Part model, mm, in its own coordinate system. A direction names the side the tool comes from. Give positions to 0.01 mm unless a question says otherwise; leave off trailing zeros. Order: outer loops, then holes, each group sorted by start corner. A loop starts at its lowest first (then second) coordinate and runs counter-clockwise, first axis right, second up.
1. Which spindle directions (+Z, -Z, +X, -X, +Y, -Y) get a long thin tool onto all of the face, cutting with end or side? Do faces 1 (the flat face through (0, 0, -12)), 2 (the cylindrical face through (14.2, 3.5, 33.2)), 3 (the flat face through (-12, -1, -44.8)). Say none if no direction does.
2. Slice it at D-D on y = -15.25. List the corners of the cut face in (x, z), and give its area (3 significant figures).
3. Drop flat-ended pins along their axis: pin 1 Ø9.5 at (x, z) = (0, -21.8) entering from -Y; pin 2 Ø5 at (x, z) = (11, 37) entering from -Y; pin 3 Ø3 at (y, z) = (-14, -47) entering from -X; pin 4 Ø4 at (x, y) = (1, -10.5) entering from +Z. Give the stop position or say it passes through.
4. Mould opens along X. For faces 4 (the cylindrical face through (-10.36, 3.52, 38.03)), 5 (the flat face through (12, -1, -44.8)), 6 (the flat face through (31.467, -1, 5)) say: +X half, -X half, draft (parallel to the pull), parting line (faces both ways), or undercut.
5. Slice it at B-B on x = -1.5. List the corners of the cut face in (y, z), and give its area (3 significant figures).
6. Slice it at C-C on x = 17.5. List the corners of the cut face in (y, z).
7. Probe line 1 (X direction, y = -2.1, z = -21.8); line 2 (Y direction, x = 17, z = -35.5); line 3 (Z direction, x = -6.5, y = -1.25). List the from-to ranges inside material, lowest first.
8. Slice it at A-A on z = -21.8. List the corners of the cut face in (x, y), and give its area (3 significant figures).
from build123d import *

# Parameters (mm, degrees)
BASE_FLANGE1_DEPTH           = 3
SKETCH2_R                    = 8
CUT_EXTRUDE1_DEPTH           = 73.112420355
EDGE_FLANGE1_STRIP_W         = 13.4732
EDGE_FLANGE1_STRIP_H         = 3
EDGE_FLANGE1_STRIP_CUT_DEPTH = 62.933077126
EDGE_FLANGE1_DEPTH           = 62.933077126
EDGE_FLANGE2_STRIP_W         = 13.4732
EDGE_FLANGE2_STRIP_H         = 3
EDGE_FLANGE2_STRIP_CUT_DEPTH = 62.933077126
EDGE_FLANGE2_DEPTH           = 62.933077126
CUT_EXTRUDE14_DEPTH          = 73.492766325
CUT_EXTRUDE15_DEPTH          = 73.492766325
CUT_EXTRUDE16_DEPTH          = 73.492766325
SKETCHED_START               = -2.498589927
SKETCHED_BEND2_DEPTH         = 5
SKETCHED_BEND2_2_DEPTH       = 5


# Read off the part's stored shape, not the designer's step: Sketched Bend2
# Sheet-metal steps are written as plain solids
with BuildPart() as part:
    # Sketch1 → Base-Flange1 (new body)
    with BuildSketch(Plane(origin=(0, 0, 0), x_dir=(1, 0, 0), z_dir=(0, 1, 0))):
        with BuildLine():
            Line((2.501410073, 64.8), (-2.498589927, 64.8))
            Line((-2.498589927, 64.8), (-2.498589927, 44.8))
            Line((-2.498589927, 44.8), (-21.498589927, 44.8))
            ThreePointArc((-21.498589927, 44.8), (-28.847059156, 41.582329983), (-31.466538563, 34))
            Line((-31.466538563, 34), (-31.466538563, -26))
            Line((-31.466538563, -26), (31.466538563, -26))
            Line((31.466538563, -26), (31.466538563, 34))
            ThreePointArc((31.466538563, 34), (28.848015597, 41.581293991), (21.501410073, 44.8))
            Line((21.501410073, 44.8), (2.501410073, 44.8))
            Line((2.501410073, 44.8), (2.501410073, 64.8))
        make_face()
    extrude(amount=-BASE_FLANGE1_DEPTH)

    # Sketch2 → Cut-Extrude1 (cut, through all)
    with BuildSketch(Plane(origin=(0, 0, 0), x_dir=(1, 0, 0), z_dir=(0, 1, 0))):
        with Locations(Location((0.000474376, 21.8, 0), (0, 0, 270))):
            Circle(SKETCH2_R)
    extrude(amount=-CUT_EXTRUDE1_DEPTH, mode=Mode.SUBTRACT)

    # Edge-Flange1 strip (across the edge) → Edge-Flange1 strip cut (cut)
    with BuildSketch(Plane(origin=(-31.466538563, 0, 26), x_dir=(0, 0, -1), z_dir=(1, 0, 0))):
        with Locations((-3, -1.5)):
            Rectangle(EDGE_FLANGE1_STRIP_W, EDGE_FLANGE1_STRIP_H)
    extrude(amount=EDGE_FLANGE1_STRIP_CUT_DEPTH, mode=Mode.SUBTRACT)

    # Edge-Flange1 section (across the edge) → Edge-Flange1 (add)
    with BuildSketch(Plane(origin=(-31.466538563, 0, 26), x_dir=(0, 0, -1), z_dir=(1, 0, 0))):
        with BuildLine():
            Line((0, 0.7366), (0, 2))
            Line((0, 2), (3, 2))
            Line((3, 2), (3, 0.7366))
            ThreePointArc((3, 0.7366), (3.215745145, 0.215745145), (3.7366, 0))
            Line((3.7366, 0), (3.7366, -3))
            ThreePointArc((3.7366, -3), (1.094424801, -1.905575199), (0, 0.7366))
        make_face()
    extrude(amount=EDGE_FLANGE1_DEPTH)

    # Edge-Flange2 strip (across the edge) → Edge-Flange2 strip cut (cut)
    with BuildSketch(Plane(origin=(31.466538563, 2, 26), x_dir=(0, -1, 0), z_dir=(-1, 0, 0))):
        with Locations((-6, -1.5)):
            Rectangle(EDGE_FLANGE2_STRIP_W, EDGE_FLANGE2_STRIP_H)
    extrude(amount=EDGE_FLANGE2_STRIP_CUT_DEPTH, mode=Mode.SUBTRACT)

    # Edge-Flange2 section (across the edge) → Edge-Flange2 (add)
    with BuildSketch(Plane(origin=(31.466538563, 2, 26), x_dir=(0, -1, 0), z_dir=(-1, 0, 0))):
        with BuildLine():
            Line((-3, 0.7366), (-3, 17))
            Line((-3, 17), (0, 17))
            Line((0, 17), (0, 0.7366))
            ThreePointArc((0, 0.7366), (0.215745145, 0.215745145), (0.7366, 0))
            Line((0.7366, 0), (0.7366, -3))
            ThreePointArc((0.7366, -3), (-1.905575199, -1.905575199), (-3, 0.7366))
        make_face()
    extrude(amount=EDGE_FLANGE2_DEPTH)

    # Sketch10 → Cut-Extrude14 (cut, through all)
    with BuildSketch(Plane(origin=(0, 5, 0), x_dir=(1, 0, 0), z_dir=(0, 1, 0))):
        with BuildLine():
            ThreePointArc((-27.999525624, -27.986488127), (-14.471973254, -33.456154948), (0, -35.319999998))
            ThreePointArc((0, -35.319999998), (14.426900142, -33.134483917), (27.829351114, -27.3650614))
            ThreePointArc((27.829351114, -27.3650614), (29.363428756, -28.706266155), (29.310299494, -30.743274178))
            ThreePointArc((29.310299494, -30.743274178), (26.455644788, -32.304474337), (23.521539899, -33.71068482))
            ThreePointArc((23.521539899, -33.71068482), (12.036275705, -37.463802008), (0.039934977, -38.907751924))
            ThreePointArc((0.039934977, -38.907751924), (-11.985574487, -37.731187287), (-23.551533984, -34.234651411))
            ThreePointArc((-23.551533984, -34.234651411), (-26.516212861, -32.894099815), (-29.404911166, -31.396828455))
            ThreePointArc((-29.404911166, -31.396828455), (-29.503369191, -29.361507737), (-27.999525624, -27.986488127))
        make_face()
    extrude(amount=-CUT_EXTRUDE14_DEPTH, mode=Mode.SUBTRACT)

    # Sketch12 → Cut-Extrude15 (cut, through all)
    with BuildSketch(Plane(origin=(0, 5, 0), x_dir=(1, 0, 0), z_dir=(0, 1, 0))):
        with BuildLine():
            Line((-7.914237019, -39.945550294), (7.914237019, -39.945550294))
            add(Edge.make_bspline(
                [(7.914237019, -39.945550294), (8.930869278, -39.730893974), (8.872112241, -38.554022125), (9.602345878, -38.030110388)],
                knots=[0, 0, 0, 0, 1, 1, 1, 1], degree=3))
            Line((9.602345878, -38.030110388), (11.562836506, -37.624091619))
            Line((11.562836506, -37.624091619), (0, -37.916784011))
            Line((0, -37.916784011), (-11.562836506, -37.624091619))
            Line((-11.562836506, -37.624091619), (-9.602345878, -38.030110388))
            add(Edge.make_bspline(
                [(-7.914237019, -39.945550294), (-8.930869278, -39.730893974), (-8.872112241, -38.554022125), (-9.602345878, -38.030110388)],
                knots=[0, 0, 0, 0, 1, 1, 1, 1], degree=3))
        make_face()
    extrude(amount=-CUT_EXTRUDE15_DEPTH, mode=Mode.SUBTRACT)

    # Sketch13 → Cut-Extrude16 (cut, through all)
    with BuildSketch(Plane(origin=(0, 5, 0), x_dir=(1, 0, 0), z_dir=(0, 1, 0))):
        with BuildLine():
            Line((-29.503369191, -29.361507737), (-30.236500006, -31.46681125))
            ThreePointArc((-30.236500006, -31.46681125), (-30.1571885, -32.842186741), (-29.128569459, -33.758642374))
            Line((-29.128569459, -33.758642374), (-14.274829355, -38.931167152))
            add(Edge.make_bspline(
                [(-14.274829355, -38.931167152), (-13.356001391, -38.419364556), (-12.413528872, -37.83920993), (-11.311548038, -37.858876708)],
                knots=[0, 0, 0, 0, 1, 1, 1, 1], degree=3))
            Line((-11.311548038, -37.858876708), (-10.639965658, -35.930319464))
            Line((-10.639965658, -35.930319464), (-29.503369191, -29.361507737))
        make_face()
        with BuildLine():
            Line((10.639965658, -35.930319464), (11.311548038, -37.858876708))
            add(Edge.make_bspline(
                [(14.274829355, -38.931167152), (13.356001391, -38.419364556), (12.413528872, -37.83920993), (11.311548038, -37.858876708)],
                knots=[0, 0, 0, 0, 1, 1, 1, 1], degree=3))
            Line((14.274829355, -38.931167152), (29.128569459, -33.758642374))
            ThreePointArc((29.128569459, -33.758642374), (30.1571885, -32.842186741), (30.236500006, -31.46681125))
            Line((30.236500006, -31.46681125), (29.503369191, -29.361507737))
            Line((29.503369191, -29.361507737), (10.639965658, -35.930319464))
        make_face()
    extrude(amount=-CUT_EXTRUDE16_DEPTH, mode=Mode.SUBTRACT)

    # Sketched Bend2 outline → Sketched Bend2 (cut)
    with BuildSketch(Plane.YZ.offset(SKETCHED_START)):
        with BuildLine():
            ThreePointArc((0, -44.8), (-0.845704021, -47.167467001), (-3, -48.463277222))
            Line((-3, -48.463277222), (-3, -64.8))
            Line((-3, -64.8), (0, -64.8))
            Line((0, -64.8), (0, -44.8))
        make_face()
    extrude(amount=SKETCHED_BEND2_DEPTH, mode=Mode.SUBTRACT)

    # Sketched Bend2 2 outline → Sketched Bend2 2 (add)
    with BuildSketch(Plane.YZ.offset(SKETCHED_START)):
        with BuildLine():
            ThreePointArc((-3, -44.8), (-3.215745145, -45.320854855), (-3.7366, -45.5366))
            Line((-3.7366, -45.5366), (-20.223356935, -45.5366))
            Line((-20.223356935, -45.5366), (-20.223356935, -48.5366))
            Line((-20.223356935, -48.5366), (-3.7366, -48.5366))
            ThreePointArc((-3.7366, -48.5366), (-3.36647982, -48.518224121), (-3, -48.463277222))
            Line((-3, -48.463277222), (-3, -44.8))
        make_face()
    extrude(amount=SKETCHED_BEND2_2_DEPTH)


solid = part.part
Data:
1. face 1: -Z, +X, -X, +Y
1. face 2: +Y, -Y
1. face 3: -Z, -X, +Y, -Y
2. outline: (-2.5, -48.54) - (2.5, -48.54) - (2.5, -45.54) - (-2.5, -45.54) - close
2. area: 15.0 mm2
3. pin 1: passes through
3. pin 2: stops at y = 2
3. pin 3: stops at x = -2.5
3. pin 4: stops at z = -45.54
4. face 4: undercut
4. face 5: draft
4. face 6: +X half
5. outline: (-20.22, -48.54) - (-3.74, -48.54) arc R3.74 ccw to (0, -44.8) - (0, -29.66) - (-3, -29.66) - (-3, -44.8) arc R0.74 cw to (-3.74, -45.54) - (-20.22, -45.54) - close; (-3, -13.94) - (0, -13.94) - (0, 22.26) arc R0.74 cw to (0.74, 23) - (1.26, 23) arc R3.74 ccw to (5, 26.74) - (5, 35.3) - (2, 35.3) - (2, 26.74) arc R0.74 cw to (1.26, 26) - (0.74, 26) arc R3.74 ccw to (-3, 22.26) - close; (2, 39.95) - (5, 39.95) - (5, 43) - (2, 43) - close
5. area: 272 mm2
6. outline: (-3, -44.8) - (0, -44.8) - (0, 22.26) arc R0.74 cw to (0.74, 23) - (1.26, 23) arc R3.74 ccw to (5, 26.74) - (5, 32.16) - (2, 32.16) - (2, 26.74) arc R0.74 cw to (1.26, 26) - (0.74, 26) arc R3.74 ccw to (-3, 22.26) - close; (2, 37.81) - (5, 37.81) - (5, 43) - (2, 43) - close
7. line 1: x = -31.47 to -8, 8 to 31.47
7. line 2: y = -3 to 0
7. line 3: z = -44.8 to -26.46, -17.14 to 25.43
8. outline: (-31.47, -3) - (-8, -3) - (-8, 0) - (-31.47, 0) - close; (8, -3) - (31.47, -3) - (31.47, 0) - (8, 0) - close
8. area: 141 mm2
